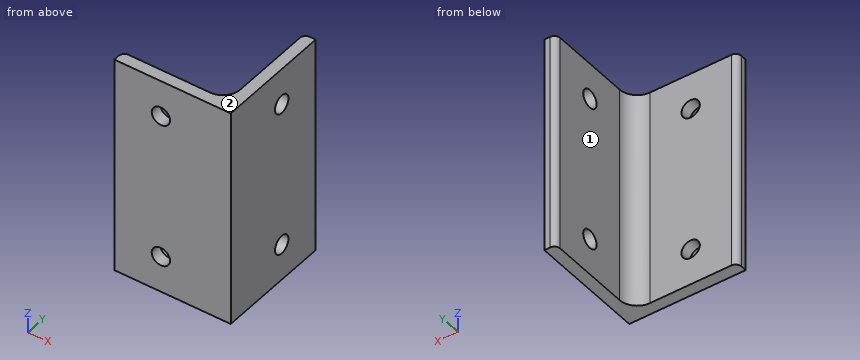
```python
from build123d import *

# Parameters (mm, degrees)
BOSS_EXTRUDE1_DEPTH = 304.8
SKETCH3_W           = 34.414454966
SKETCH3_H           = 33.657940314
CUT_EXTRUDE1_DEPTH  = 549.6
SKETCH5_R           = 2.5
CUT_EXTRUDE2_DEPTH  = 101.6
SKETCH4_R           = 2.5
CUT_EXTRUDE3_DEPTH  = 101.6


with BuildPart() as part:
    # Sketch2 → Boss-Extrude1 (new, symmetric)
    with BuildSketch(Plane.XY):
        with BuildLine():
            Line((-15.875, -15.875), (15.875, -15.875))
            Line((15.875, -15.875), (15.875, 15.875))
            Line((15.875, 15.875), (14.2875, 15.875))
            ThreePointArc((14.2875, 15.875), (13.164967985, 15.410032015), (12.7, 14.2875))
            Line((12.7, 14.2875), (12.7, -7.9248))
            ThreePointArc((12.7, -7.9248), (11.301376302, -11.301376302), (7.9248, -12.7))
            Line((7.9248, -12.7), (-14.2875, -12.7))
            ThreePointArc((-14.2875, -12.7), (-15.410032015, -13.164967985), (-15.875, -14.2875))
            Line((-15.875, -14.2875), (-15.875, -15.875))
        make_face()
    extrude(amount=BOSS_EXTRUDE1_DEPTH, both=True)

    # Sketch3 → Cut-Extrude1 (cut)
    with BuildSketch(Plane(origin=(0, 0, -304.8), x_dir=(-1, 0, 0), z_dir=(0, 0, -1))):
        with Locations((1.332227483, 0.953970157)):
            Rectangle(SKETCH3_W, SKETCH3_H)
    extrude(amount=-CUT_EXTRUDE1_DEPTH, mode=Mode.SUBTRACT)

    # Sketch5 → Cut-Extrude2 (cut)
    with BuildSketch(Plane.ZY.offset(-12.7)):
        with Locations(Location((294.8, 3.18135, 0), (0, 0, 270))):
            Circle(SKETCH5_R)
        with Locations(Location((254.8, 3.18135, 0), (0, 0, 270))):
            Circle(SKETCH5_R)
    extrude(amount=-CUT_EXTRUDE2_DEPTH, mode=Mode.SUBTRACT)

    # Sketch4 → Cut-Extrude3 (cut)
    with BuildSketch(Plane(origin=(0, -12.7, 0), x_dir=(1, 0, 0), z_dir=(0, 1, 0))):
        with Locations(Location((-3.18135, -254.8, 0), (0, 0, 180))):
            Circle(SKETCH4_R)
        with Locations(Location((-3.18135, -294.8, 0), (0, 0, 180))):
            Circle(SKETCH4_R)
    extrude(amount=-CUT_EXTRUDE3_DEPTH, mode=Mode.SUBTRACT)


solid = part.part
```
Check sheet for the modelled part. Datum: model origin and axes. Units: mm. Face numbers are marked on the shaded views. A direction names the side the tool comes from. Round coordinates to 2 decimals unless told otherwise and drop trailing zeros. Loops run counter-clockwise (first coordinate to the right, second up) from the corner with the lowest first, then second, coordinate; pieces in that order, holes last. Notation, with made-up numbers: (84, 18) -> (126, 18) arc R26 ccw to (126, 36) -> close; hole circle Ø1 at (-30.75, -30). An arc over 180 degrees is marked (long way). Write item = value, one per line. Start each with the question number.
1) Sectioned sample at C-C, the plane y = 3.5. Record the cut outline in (x, z) (3 decimals).
2) Sectioned sample at D-D, the plane z = 265.5. Record the cut outline in (x, y) (1 decimal).
3) Thickness scan on probe 1 along Y at (x, z) = (15, 294.8) (3 decimals); probe 2 along Z at (x, y) = (-2, -13); probe 3 along Y at (x, z) = (3.5, 251.5) (3 decimals). Record the ranges inside material, lowest first.
4) Sectioned sample at B-B, the plane x = -3. Record the cut outline in (y, z) (3 decimals), plus the area to 3 significant figures.
5) Set-up check for the marked faces 1 and 2: record each of +Z, -Z, +X, -X, +Y, -Y from which the full face is reachable in a straight line by a thin tool's end or side.
6) Sectioned sample at A-A, the plane z = 254.8. Record the cut outline in (x, y) (1 decimal), plus the area to 3 significant figures.
7) Gauge pin test, flat ends, axial feed: pin 1 Ø2 at (x, z) = (-7.5, 288.5) entering from +Y; pin 2 Ø4 at (y, z) = (-11.5, 266.5) entering from -X; pin 3 Ø6.5 at (y, z) = (4, 261.5) entering from -X. Record the tip position at first contact, or that the pin passes through.
Results are:
q1.outline = (12.7, 244.8) -> (15.875, 244.8) -> (15.875, 252.32) -> (12.7, 252.32) -> close; (12.7, 257.28) -> (15.875, 257.28) -> (15.875, 292.32) -> (12.7, 292.32) -> close; (12.7, 297.28) -> (15.875, 297.28) -> (15.875, 304.8) -> (12.7, 304.8) -> close
q2.outline = (-15.9, -15.9) -> (15.9, -15.9) -> (15.9, 15.9) -> (14.3, 15.9) arc R1.6 ccw to (12.7, 14.3) -> (12.7, -7.9) arc R4.8 cw to (7.9, -12.7) -> (-14.3, -12.7) arc R1.6 ccw to (-15.9, -14.3) -> close
q3.probe_1 = -15.875 to 0.681, 5.681 to 15.875
q3.probe_2 = 244.8 to 252.6, 257 to 292.6, 297 to 304.8
q3.probe_3 = -15.875 to -12.7
q4.outline = (-15.875, 244.8) -> (-12.7, 244.8) -> (-12.7, 252.307) -> (-15.875, 252.307) -> close; (-15.875, 257.293) -> (-12.7, 257.293) -> (-12.7, 292.307) -> (-15.875, 292.307) -> close; (-15.875, 297.293) -> (-12.7, 297.293) -> (-12.7, 304.8) -> (-15.875, 304.8) -> close
q4.area = 159 mm^2
q5.face_1 = +Z, -Z, -X, +Y
q5.face_2 = +Z, +X, -X, +Y, -Y
q6.outline = (-15.9, -15.9) -> (-5.7, -15.9) -> (-5.7, -12.7) -> (-14.3, -12.7) arc R1.6 ccw to (-15.9, -14.3) -> close; (-0.7, -15.9) -> (15.9, -15.9) -> (15.9, 0.7) -> (12.7, 0.7) -> (12.7, -7.9) arc R4.8 cw to (7.9, -12.7) -> (-0.7, -12.7) -> close; (12.7, 5.7) -> (15.9, 5.7) -> (15.9, 15.9) -> (14.3, 15.9) arc R1.6 ccw to (12.7, 14.3) -> close
q6.area = 164 mm^2
q7.pin_1 = -12.7
q7.pin_2 = -15.67
q7.pin_3 = 12.7
